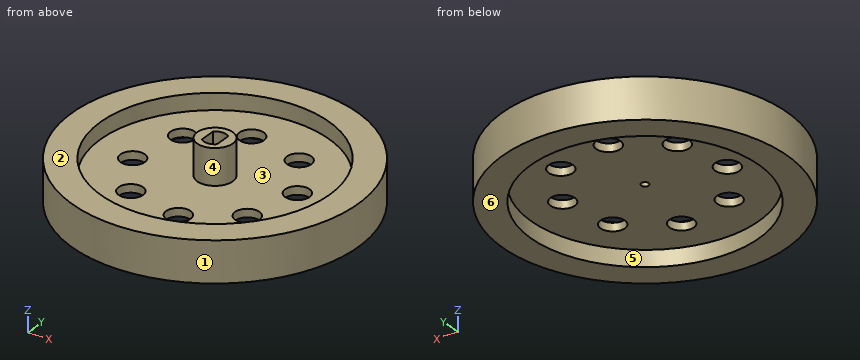
from build123d import *

# Parameters (mm, degrees)
SKETCH2_R          = 3
CUT_EXTRUDE1_DEPTH = 2
CUT_EXTRUDE2_DEPTH = 8.75
SKETCH4_R          = 0.95
CUT_EXTRUDE3_DEPTH = 2


with BuildPart() as part:
    # Sketch1 → Revolve1 (revolve)
    with BuildSketch(Plane(origin=(0, 0, 0), x_dir=(0, 0, -1), z_dir=(1, 0, 0))):
        Polygon((0, 0), (-9.75, 0), (-9.75, 4.367299354), (-1, 4.367299354), (-1, 28), (-5, 28), (-5, 35), (5, 35), (5, 28), (1, 28), (1, 0), align=None)
    revolve(axis=Axis((0, 0, 0), (0, 0, 1)))

    # Sketch2 → Cut-Extrude1 (cut)
    with BuildSketch(Plane(origin=(0, 0, -1), x_dir=(-1, 0, 0), z_dir=(0, 0, -1))):
        with Locations((-10.543910988, 15)):
            Circle(SKETCH2_R)
        with Locations((3.150930758, 18.062272677)):
            Circle(SKETCH2_R)
        with Locations((15, 10.543910988)):
            Circle(SKETCH2_R)
        with Locations((18.062272677, -3.150930758)):
            Circle(SKETCH2_R)
        with Locations((10.543910988, -15)):
            Circle(SKETCH2_R)
        with Locations((-3.150930758, -18.062272677)):
            Circle(SKETCH2_R)
        with Locations((-15, -10.543910988)):
            Circle(SKETCH2_R)
        with Locations((-18.062272677, 3.150930758)):
            Circle(SKETCH2_R)
    extrude(amount=-CUT_EXTRUDE1_DEPTH, mode=Mode.SUBTRACT)

    # Sketch3 → Cut-Extrude2 (cut)
    with BuildSketch(Plane.XY.offset(9.75)):
        with BuildLine():
            Line((1.85, -2.034698995), (1.85, 2.034698995))
            ThreePointArc((1.85, 2.034698995), (0, 2.75), (-1.85, 2.034698995))
            Line((-1.85, 2.034698995), (-1.85, -2.034698995))
            ThreePointArc((-1.85, -2.034698995), (0, -2.75), (1.85, -2.034698995))
        make_face()
    extrude(amount=-CUT_EXTRUDE2_DEPTH, mode=Mode.SUBTRACT)

    # Sketch4 → Cut-Extrude3 (cut)
    with BuildSketch(Plane(origin=(0, 0, -1), x_dir=(-1, 0, 0), z_dir=(0, 0, -1))):
        Circle(SKETCH4_R)
    extrude(amount=-CUT_EXTRUDE3_DEPTH, mode=Mode.SUBTRACT)


solid = part.part
Read the model definition and answer for the solid it produces. Units are mm, in the model's axes. Face numbers are marked on the shaded views. A direction names the side the tool comes from. Give positions to 0.01 mm unless a question says otherwise; leave off trailing zeros. Loops run counter-clockwise (first coordinate to the right, second up) from the corner with the lowest first, then second, coordinate; pieces in that order, holes last. Notation, with made-up numbers: (37.5, 49.5) -> (91.5, 49.5) arc R7 cw to (91.5, 53.5) -> close; hole circle Ø5 at (70.25, 50.25). An arc over 180 degrees is marked (long way). Use a Markdown table: item, result.
Q1. Section A-A, the plane y = -16.5 is taken. Determine the outline of the cut face in (x, z).
Solved:
| item | result |
|---|---|
| outline | (-30.87, -5) -> (-22.62, -5) -> (-22.62, -1) -> (-13.14, -1) -> (-13.14, 1) -> (-22.62, 1) -> (-22.62, 5) -> (-30.87, 5) -> close; (-7.95, -1) -> (0.59, -1) -> (0.59, 1) -> (-7.95, 1) -> close; (5.71, -1) -> (22.62, -1) -> (22.62, -5) -> (30.87, -5) -> (30.87, 5) -> (22.62, 5) -> (22.62, 1) -> (5.71, 1) -> close |
Q2. Find the intervals of material crossed by line 1 along Z through (x, y) = (-22, -15.5); line 2 along Y through (x, z) = (19.5, -4); line 3 along Y through (x, z) = (0, 0.2), in increasing order.
Solved:
| item | result |
|---|---|
| line 1 | z = -1 to 1 |
| line 2 | y = -29.06 to -20.09, 20.09 to 29.06 |
| line 3 | y = -35 to -0.95, 0.95 to 35 |
Q3. Each of these flat-tipped pins is pushed along its axis until it touches: pin 1 (7 mm diameter, centred on x = -3.15, y = 18.06, fed in from -Z); pin 2 (3 mm diameter, centred on x = 13.5, z = 2.5, fed in from +Y); pin 3 (2 mm diameter, centred on y = -1, z = 7.5, fed in from +X); pin 4 (5.5 mm diameter, centred on x = -15, y = 10.54, fed in from -Z). Where does it stop, or does it pass through?
Solved:
| item | result |
|---|---|
| pin 1 | stops at z = -1 |
| pin 2 | stops at y = 32.88 |
| pin 3 | stops at x = 4.37 |
| pin 4 | passes through |
Q4. A tool of negligible diameter and unlimited length cuts with its end or side. For the marked faces 4, 5 and 6, from which of +Z, -Z, +X, -X, +Y, -Y can it reach the whole face along a straight path? Write none if from no direction.
Solved:
| item | result |
|---|---|
| face 4 | +Z |
| face 5 | -Z |
| face 6 | -Z, +X, -X, +Y, -Y |
Q5. Determine the mould class of the marked faces 1, 2 and 3 for opening direction Y: pulls with the +Y half, pulls with the -Y half, needs draft (parallel to the pull), parting line crosses it, or undercut.
Solved:
| item | result |
|---|---|
| face 1 | parting line crosses it |
| face 2 | needs draft |
| face 3 | undercut |
Q6. Section B-B, the plane x = -25.5 is taken. Determine the outline of the cut face in (y, z), then the cut area to 3 significant figures.
Solved:
| item | result |
|---|---|
| outline | (-23.97, -5) -> (-11.57, -5) -> (-11.57, -1) -> (11.57, -1) -> (11.57, -5) -> (23.97, -5) -> (23.97, 5) -> (11.57, 5) -> (11.57, 1) -> (-11.57, 1) -> (-11.57, 5) -> (-23.97, 5) -> close |
| area | 294 mm^2 |
